from build123d import *

# Parameters (mm, degrees)
ESQUISSE1_R             = 1.5
ESQUISSE1_W             = 4
ESQUISSE1_H             = 7
ESQUISSE1_W_2           = 6
ESQUISSE1_H_2           = 4
BOSS_EXTRU_1_DEPTH      = 4
ENL_V_MAT_EXTRU_1_REACH = 59.99
ENL_V_MAT_EXTRU_2_REACH = 59.99
ENL_V_MAT_EXTRU_3_REACH = 59.99
CONG_1_R                = 3.5
CONG_2_R                = 3.5
CONG_3_R                = 1.5
ENL_V_MAT_EXTRU_4_REACH = 59.99
CONG_4_R                = 3
CONG_5_R                = 3
ENL_V_MAT_EXTRU_5_REACH = 59.99
ESQUISSE8_R             = 3.5
CONG_6_R                = 1.5
ENL_V_MAT_EXTRU_6_REACH = 59.99
ESQUISSE9_R             = 1.5


with BuildPart() as part:
    # Esquisse1 → Boss.-Extru.1 (new body)
    with BuildSketch(Plane(origin=(0, 0, 0), x_dir=(1, 0, 0), z_dir=(0, 1, 0))):
        Polygon((-20.28, 5), (-22.28, 5), (-22.28, -37), (-34.66, -37), (-34.66, -46.32), (34.66, -46.32), (34.66, -37), (22.28, -37), (22.28, 5), (20.28, 5), (16.28, 5), (16.28, 13), (5, 13), (5, 35), (-5, 35), (-5, 13), (-16.28, 13), (-16.28, 5), align=None)
        with Locations(Location((-5, 0, 0), (0, 0, 270))):
            Circle(ESQUISSE1_R, mode=Mode.SUBTRACT)
        with Locations(Location((5, 0, 0), (0, 0, 90))):
            Circle(ESQUISSE1_R, mode=Mode.SUBTRACT)
        with Locations(Location((-30, -41.66, 0), (0, 0, 270))):
            Circle(ESQUISSE1_R, mode=Mode.SUBTRACT)
        with Locations(Location((30, -41.66, 0), (0, 0, 90))):
            Circle(ESQUISSE1_R, mode=Mode.SUBTRACT)
        with Locations((0, 27.42)):
            Rectangle(ESQUISSE1_W, ESQUISSE1_H, mode=Mode.SUBTRACT)
        with Locations((-17.5, -13.5)):
            Rectangle(ESQUISSE1_W, ESQUISSE1_H, mode=Mode.SUBTRACT)
        with Locations((-7, -38.16)):
            Rectangle(ESQUISSE1_W_2, ESQUISSE1_H_2, mode=Mode.SUBTRACT)
        with Locations((7, -38.16)):
            Rectangle(ESQUISSE1_W_2, ESQUISSE1_H_2, mode=Mode.SUBTRACT)
        with Locations((17.5, -13.5)):
            Rectangle(ESQUISSE1_W, ESQUISSE1_H, mode=Mode.SUBTRACT)
    extrude(amount=BOSS_EXTRU_1_DEPTH)

    # Esquisse2 → Enlèv. mat.-Extru.1 (cut, up to next)
    with BuildSketch(Plane(origin=(0, 4, 0), x_dir=(1, 0, 0), z_dir=(0, 1, 0)), mode=Mode.PRIVATE) as enl_v_mat_extru_1_sk1:
        with BuildLine():
            ThreePointArc((-14.9974668, -7.843519448), (-14.058937243, -8.627559279), (-13.321584394, -9.603195975))
            ThreePointArc((-13.321584394, -9.603195975), (-12.428040198, -10.235555734), (-11.361521034, -9.988904221))
            ThreePointArc((-11.361521034, -9.988904221), (-8.447920047, -8.097394436), (-5.290042477, -6.650090308))
            ThreePointArc((-5.290042477, -6.650090308), (-4.088898303, -4.755535803), (-5.589901119, -3.088480121))
            ThreePointArc((-5.589901119, -3.088480121), (-7.276914991, -2.168490468), (-8.113566287, -0.438631695))
            ThreePointArc((-8.113566287, -0.438631695), (-9.70546362, 1.141857781), (-11.656322949, 0.034504187))
            ThreePointArc((-11.656322949, 0.034504187), (-13.25585737, -3.049060247), (-15.287160414, -5.866982872))
            ThreePointArc((-15.287160414, -5.866982872), (-15.585513038, -6.920209252), (-14.9974668, -7.843519448))
        make_face()
    enl_v_mat_extru_1_tool1 = extrude(enl_v_mat_extru_1_sk1.sketch, amount=-ENL_V_MAT_EXTRU_1_REACH, mode=Mode.PRIVATE) & part.part
    # Esquisse2 → Enlèv. mat.-Extru.1 (cut, up to next)
    with BuildSketch(Plane(origin=(0, 4, 0), x_dir=(1, 0, 0), z_dir=(0, 1, 0)), mode=Mode.PRIVATE) as enl_v_mat_extru_1_sk2:
        with BuildLine():
            ThreePointArc((5.589901119, -3.088480121), (4.088898303, -4.755535803), (5.290042477, -6.650090308))
            ThreePointArc((5.290042477, -6.650090308), (8.447920047, -8.097394436), (11.361521034, -9.988904221))
            ThreePointArc((11.361521034, -9.988904221), (12.428040198, -10.235555734), (13.321584394, -9.603195975))
            ThreePointArc((13.321584394, -9.603195975), (14.058937243, -8.627559279), (14.9974668, -7.843519448))
            ThreePointArc((14.9974668, -7.843519448), (15.585513038, -6.920209252), (15.287160414, -5.866982872))
            ThreePointArc((15.287160414, -5.866982872), (13.25585737, -3.049060247), (11.656322949, 0.034504187))
            ThreePointArc((11.656322949, 0.034504187), (9.70546362, 1.141857781), (8.113566287, -0.438631695))
            ThreePointArc((8.113566287, -0.438631695), (7.276914991, -2.168490468), (5.589901119, -3.088480121))
        make_face()
    enl_v_mat_extru_1_tool2 = extrude(enl_v_mat_extru_1_sk2.sketch, amount=-ENL_V_MAT_EXTRU_1_REACH, mode=Mode.PRIVATE) & part.part
    add(enl_v_mat_extru_1_tool1.solids().sort_by_distance((-10.104676, 4, 4.861596))[0], mode=Mode.SUBTRACT)
    add(enl_v_mat_extru_1_tool2.solids().sort_by_distance((10.104676, 4, 4.861596))[0], mode=Mode.SUBTRACT)

    # Esquisse3 → Enlèv. mat.-Extru.2 (cut, up to next)
    with BuildSketch(Plane(origin=(0, 4, 0), x_dir=(1, 0, 0), z_dir=(0, 1, 0)), mode=Mode.PRIVATE) as enl_v_mat_extru_2_sk1:
        with BuildLine():
            ThreePointArc((-3.934570919, -34.661427668), (-3.25, -34.860961894), (-2.734912831, -35.354050587))
            ThreePointArc((-2.734912831, -35.354050587), (-1.93927123, -36.028172694), (-0.901821799, -36.133931151))
            ThreePointArc((-0.901821799, -36.133931151), (0, -36.043871504), (0.901821799, -36.133931151))
            ThreePointArc((0.901821799, -36.133931151), (1.93927123, -36.028172694), (2.734912831, -35.354050587))
            ThreePointArc((2.734912831, -35.354050587), (3.25, -34.860961894), (3.934570919, -34.661427668))
            ThreePointArc((3.934570919, -34.661427668), (7.745395438, -30.322645486), (3.25, -26.697892503))
            ThreePointArc((3.25, -26.697892503), (0, -26.90596734), (-3.25, -26.697892503))
            ThreePointArc((-3.25, -26.697892503), (-7.745395438, -30.322645486), (-3.934570919, -34.661427668))
        make_face()
    enl_v_mat_extru_2_tool1 = extrude(enl_v_mat_extru_2_sk1.sketch, amount=-ENL_V_MAT_EXTRU_2_REACH, mode=Mode.PRIVATE) & part.part
    add(enl_v_mat_extru_2_tool1.solids().sort_by_distance((0, 4, 31.014004))[0], mode=Mode.SUBTRACT)

    # Esquisse4 → Enlèv. mat.-Extru.3 (cut, up to next)
    with BuildSketch(Plane(origin=(0, 4, 0), x_dir=(1, 0, 0), z_dir=(0, 1, 0)), mode=Mode.PRIVATE) as enl_v_mat_extru_3_sk1:
        with BuildLine():
            ThreePointArc((-1.504993876, -23.185356229), (0, -23.237327603), (1.504993876, -23.185356229))
            ThreePointArc((1.504993876, -23.185356229), (2.895700447, -23.245383622), (4.238200501, -23.613298912))
            ThreePointArc((4.238200501, -23.613298912), (5.947114761, -23.612368685), (7.184676805, -22.433882792))
            ThreePointArc((7.184676805, -22.433882792), (7.833923694, -20.976940348), (8.452629907, -19.506768443))
            ThreePointArc((8.452629907, -19.506768443), (8.650133896, -14.04633429), (5.268411363, -9.754562897))
            ThreePointArc((5.268411363, -9.754562897), (4.141434744, -9.367776338), (2.957336552, -9.500409716))
            ThreePointArc((2.957336552, -9.500409716), (0, -9.996838884), (-2.957336552, -9.500409716))
            ThreePointArc((-2.957336552, -9.500409716), (-4.141434744, -9.367776338), (-5.268411363, -9.754562897))
            ThreePointArc((-5.268411363, -9.754562897), (-8.650133896, -14.04633429), (-8.452629907, -19.506768443))
            ThreePointArc((-8.452629907, -19.506768443), (-7.833923694, -20.976940348), (-7.184676805, -22.433882792))
            ThreePointArc((-7.184676805, -22.433882792), (-5.947114761, -23.612368685), (-4.238200501, -23.613298912))
            ThreePointArc((-4.238200501, -23.613298912), (-2.895700447, -23.245383622), (-1.504993876, -23.185356229))
        make_face()
    enl_v_mat_extru_3_tool1 = extrude(enl_v_mat_extru_3_sk1.sketch, amount=-ENL_V_MAT_EXTRU_3_REACH, mode=Mode.PRIVATE) & part.part
    add(enl_v_mat_extru_3_tool1.solids().sort_by_distance((0, 4, 16.621533))[0], mode=Mode.SUBTRACT)

    # Congé1
    cong_1_edges = [part.edges().sort_by_distance(p)[0] for p in [
        (-5, 2, -35),
        (5, 2, -35),
    ]]
    fillet(cong_1_edges, radius=CONG_1_R)

    # Congé2
    cong_2_edges = [part.edges().sort_by_distance(p)[0] for p in [
        (-5, 2, -13),
        (5, 2, -13),
    ]]
    fillet(cong_2_edges, radius=CONG_2_R)

    # Congé3
    cong_3_edges = [part.edges().sort_by_distance(p)[0] for p in [
        (22.28, 2, -5),
        (-22.28, 2, -5),
        (-16.28, 2, -13),
        (16.28, 2, -13),
    ]]
    fillet(cong_3_edges, radius=CONG_3_R)

    # Esquisse7 → Enlèv. mat.-Extru.4 (cut, up to next)
    with BuildSketch(Plane(origin=(0, 4, 0), x_dir=(1, 0, 0), z_dir=(0, 1, 0)), mode=Mode.PRIVATE) as enl_v_mat_extru_4_sk1:
        with BuildLine():
            Line((-22.28, -17), (-22.28, -37))
            ThreePointArc((-22.28, -37), (-16.000012961, -35.267986448), (-11.495708343, -30.561677059))
            ThreePointArc((-11.495708343, -30.561677059), (-11.263143502, -24.222708134), (-16.146891575, -20.174792843))
            ThreePointArc((-16.146891575, -20.174792843), (-17.81186512, -19.879037913), (-19.5, -19.78))
            ThreePointArc((-19.5, -19.78), (-21.465756852, -18.965756852), (-22.28, -17))
        make_face()
    enl_v_mat_extru_4_tool1 = extrude(enl_v_mat_extru_4_sk1.sketch, amount=-ENL_V_MAT_EXTRU_4_REACH, mode=Mode.PRIVATE) & part.part
    enl_v_mat_extru_4 = enl_v_mat_extru_4_tool1.solids().sort_by_distance((-17.328715, 4, 27.806477))[0]
    add(enl_v_mat_extru_4, mode=Mode.SUBTRACT)

    # Symétrie1: Enlèv. mat.-Extru.4 across plane
    add(enl_v_mat_extru_4.mirror(Plane(origin=(0, 0, 0), x_dir=(0, 0, 1), z_dir=(1, 0, 0))), mode=Mode.SUBTRACT)

    # Congé4
    cong_4_edges = [part.edges().sort_by_distance(p)[0] for p in [
        (-34.66, 2, 46.32),
        (-34.66, 2, 37),
    ]]
    fillet(cong_4_edges, radius=CONG_4_R)

    # Congé5
    cong_5_edges = [part.edges().sort_by_distance(p)[0] for p in [
        (34.66, 2, 37),
        (34.66, 2, 46.32),
    ]]
    fillet(cong_5_edges, radius=CONG_5_R)

    # Esquisse8 → Enlèv. mat.-Extru.5 (cut, up to next)
    with BuildSketch(Plane(origin=(0, 4, 0), x_dir=(1, 0, 0), z_dir=(0, 1, 0)), mode=Mode.PRIVATE) as enl_v_mat_extru_5_sk1:
        with Locations((-15, -46.32)):
            Circle(ESQUISSE8_R)
    enl_v_mat_extru_5_tool1 = extrude(enl_v_mat_extru_5_sk1.sketch, amount=-ENL_V_MAT_EXTRU_5_REACH, mode=Mode.PRIVATE) & part.part
    # Esquisse8 → Enlèv. mat.-Extru.5 (cut, up to next)
    with BuildSketch(Plane(origin=(0, 4, 0), x_dir=(1, 0, 0), z_dir=(0, 1, 0)), mode=Mode.PRIVATE) as enl_v_mat_extru_5_sk2:
        with Locations((15, -46.32)):
            Circle(ESQUISSE8_R)
    enl_v_mat_extru_5_tool2 = extrude(enl_v_mat_extru_5_sk2.sketch, amount=-ENL_V_MAT_EXTRU_5_REACH, mode=Mode.PRIVATE) & part.part
    add(enl_v_mat_extru_5_tool1.solids().sort_by_distance((-15, 4, 46.32))[0], mode=Mode.SUBTRACT)
    add(enl_v_mat_extru_5_tool2.solids().sort_by_distance((15, 4, 46.32))[0], mode=Mode.SUBTRACT)

    # Congé6
    cong_6_edges = [part.edges().sort_by_distance(p)[0] for p in [
        (-18.5, 2, 46.32),
        (-11.5, 2, 46.32),
        (11.5, 2, 46.32),
        (18.5, 2, 46.32),
    ]]
    fillet(cong_6_edges, radius=CONG_6_R)

    # Esquisse9 → Enlèv. mat.-Extru.6 (cut, up to next)
    with BuildSketch(Plane(origin=(0, 4, 0), x_dir=(1, 0, 0), z_dir=(0, 1, 0)), mode=Mode.PRIVATE) as enl_v_mat_extru_6_sk1:
        with Locations(Location((-18.609395269, -40.077557629, 0), (0, 0, 270))):
            Circle(ESQUISSE9_R)
    enl_v_mat_extru_6_tool1 = extrude(enl_v_mat_extru_6_sk1.sketch, amount=-ENL_V_MAT_EXTRU_6_REACH, mode=Mode.PRIVATE) & part.part
    enl_v_mat_extru_6 = enl_v_mat_extru_6_tool1.solids().sort_by_distance((-18.609395, 4, 40.077558))[0]
    add(enl_v_mat_extru_6, mode=Mode.SUBTRACT)

    # Symétrie2: Enlèv. mat.-Extru.6 across plane
    add(enl_v_mat_extru_6.mirror(Plane(origin=(0, 0, 0), x_dir=(0, 0, 1), z_dir=(1, 0, 0))), mode=Mode.SUBTRACT)


solid = part.part
Part model, mm, in its own coordinate system. A direction names the side the tool comes from. Round coordinates to 2 decimals unless told otherwise and drop trailing zeros. Loops run counter-clockwise (first coordinate to the right, second up) from the corner with the lowest first, then second, coordinate; pieces in that order, holes last. Notation, with made-up numbers: (17, 88) - (53, 88) arc R15 cw to (53, 103) - close; hole circle Ø5 at (41.5, -10). An arc over 180 degrees is marked (long way). Answer as a JSON object with one key per item and string values.
Item 1: Band-saw the part on A-A on x = 30. List the corners of the cut face in (y, z).
Output:
{"outline": "(0, 37) - (4, 37) - (4, 40.16) - (0, 40.16) - close; (0, 43.16) - (4, 43.16) - (4, 46.32) - (0, 46.32) - close"}
Item 2: Band-saw the part on C-C on z = 11.5. List the corners of the cut face in (x, y), plus the area to 3 significant figures.
Output:
{"outline": "(-22.28, 0) - (-19.5, 0) - (-19.5, 4) - (-22.28, 4) - close; (-15.5, 0) - (-7.26, 0) - (-7.26, 4) - (-15.5, 4) - close; (7.26, 0) - (15.5, 0) - (15.5, 4) - (7.26, 4) - close; (19.5, 0) - (22.28, 0) - (22.28, 4) - (19.5, 4) - close", "area": "88.2 mm2"}
Item 3: Pull direction X, two halves, no side cores. Call faces 1 (the face through (-12.444, 2.028, 10.232)), 2 (the face through (-12, 2, -13)), 3 (the face through (16.28, 2, -8)): pulls with the +X half, pulls with the -X half, needs draft (parallel to the pull), parting line crosses it, or undercut.
Output:
{"face 1": "undercut", "face 2": "needs draft", "face 3": "pulls with the +X half"}
Item 4: Pin check, flat tips, straight feed: pin 1 (1.2 mm diameter, centred on y = 1.5, z = 13, fed in from -X); pin 2 (2 mm diameter, centred on x = -18, y = 2, fed in from -Z); pin 3 (1.2 mm diameter, centred on y = 2.5, z = 38, fed in from +X); pin 4 (2.5 mm diameter, centred on x = -18.61, z = 40.08, fed in from +Y). Stop position of each tip, or through.
Output:
{"pin 1": "x = -22.28", "pin 2": "z = -5", "pin 3": "x = 34.31", "pin 4": "through"}
Item 5: Wall check: L1, parallel to X at y = 2, z = 41.66; L2, parallel to X at y = 0.4, z = 40; L3, parallel to X at y = 3.05, z = -26. Give the ranges that are in metal, low to high.
Output:
{"L1": "-34.66 to -31.5, -28.5 to 28.5, 31.5 to 34.66", "L2": "-34.66 to -20.11, -17.11 to -10, -4 to 4, 10 to 17.11, 20.11 to 34.66", "L3": "-5 to -2, 2 to 5"}
Item 6: Band-saw the part on B-B on z = -28. List the corners of the cut face in (x, y), plus the area to 3 significant figures.
Output:
{"outline": "(-5, 0) - (-2, 0) - (-2, 4) - (-5, 4) - close; (2, 0) - (5, 0) - (5, 4) - (2, 4) - close", "area": "24.0 mm2"}
Item 7: Band-saw the part on D-D on y = 0.95. State how many separate pieces and enclosed holes the cut face has, plus the area to 3 significant figures.
Output:
{"separate pieces": "1", "enclosed holes": "15", "area": "1,960 mm2"}
Item 8: Tool access for faces 4 (the face through (-21.44, 2.03, 18.99)), 5 (the face through (22.28, 2, 7)), 6 (the face through (-33.76, 2.03, 45.46)), 7 (the face through (-8.49, 2.03, 8.12)): list every direction of +Z, -Z, +X, -X, +Y, -Y with a clear straight run to the whole face (end or side of a thin tool).
Output:
{"face 4": "-X, +Y, -Y", "face 5": "-Z, +X, +Y, -Y", "face 6": "+Z, -X, +Y, -Y", "face 7": "+Y, -Y"}
